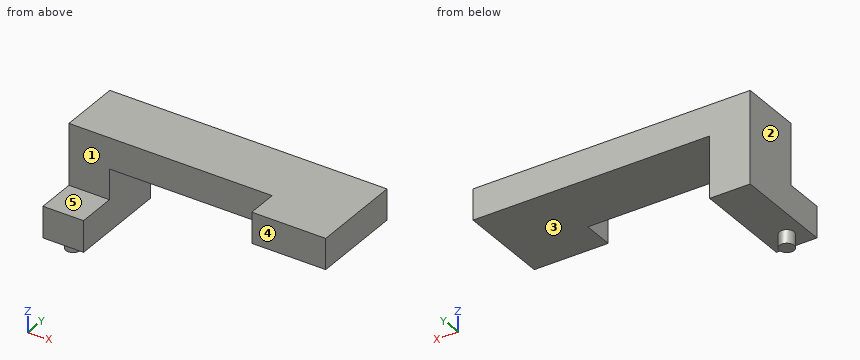
from build123d import *

# Parameters (mm, degrees)
F1_DEPTH = 25.4
F2_W     = 16.7198777199
F2_H     = 12.9023268819
F3_DEPTH = 16.1335784942
F5_W     = 30.4973670125
F5_H     = 12.7
F6_DEPTH = 12.7
F7_R     = 3.015717516
F8_DEPTH = 18.4404


with BuildPart() as f1:
    # F0 (on Front) → F1 (new body)
    with BuildSketch(Plane.XZ):
        Polygon((57.6506801724, -27.7302754164), (-56.6493198276, -27.7302754164), (-56.6493198276, -65.8302754164), (-39.9294421077, -65.8302754164), (-39.9294421077, -40.4302754164), (57.6506801724, -40.4302754164), align=None)
    extrude(amount=F1_DEPTH)

    # F2 (on face) → F3 (join)
    with BuildSketch(Plane.XZ.offset(25.4)):
        with Locations((-48.2893809676, -59.3791119754)):
            Rectangle(F2_W, F2_H)
    extrude(amount=F3_DEPTH)

    # F5 (on face) → F6 (join)
    with BuildSketch(Plane.XZ.offset(25.4)):
        with Locations((42.4019966662, -34.0802754164)):
            Rectangle(F5_W, F5_H)
    extrude(amount=F6_DEPTH)

    # F7 (on face) → F8 (join)
    with BuildSketch(Plane.XY.offset(-52.9279485345)):
        with Locations((-49.315456301, -33.8529422879)):
            Circle(F7_R)
    extrude(amount=-F8_DEPTH)


solid = f1.part
Design review of the part built by this model. Coordinates are the model's own, in mm. Face numbers are marked on the shaded views. A direction names the side the tool comes from. Round coordinates to 2 decimals unless told otherwise and drop trailing zeros. Order: outer loops, then holes, each group sorted by start corner. A loop starts at its lowest first (then second) coordinate and runs counter-clockwise, first axis right, second up. Notation, with made-up numbers: M -36,76 L -22,76 A27 cw -22,93 Z; hole C 0.25,-29.5 d10. An arc over 180 degrees is marked long. Answer as CSV lines item,"result". Start each with the question number.
1) Tool access review of the marked faces 1, 2, 3, 4 and 5: name each direction out of +Z, -Z, +X, -X, +Y, -Y from which nothing blocks a thin tool from reaching the whole face with its end or side.
2) For pin 1 Ø17.5 at (x, y) = (-48, -33.5) entering from +Z; pin 2 Ø8.5 at (x, y) = (-50.5, -10.5) entering from -Z; pin 3 Ø12.5 at (x, z) = (-10, -44.5) entering from -Y; pin 4 Ø7.5 at (y, z) = (-17.5, -53.5) entering from +X, all flat-tipped, find the tip position at first contact; note any pin that passes through.
3) Wall thickness on line 1 along Z through (x, y) = (-4.5, -13.5); line 2 along Z through (x, y) = (-43, -26); line 3 along Y through (x, z) = (-22, -37): over which ranges is each line inside the solid? List them lowest first. Write a range as [from, to].
4) Add section D-D (y = -3). Give the boundary of the cut face in (x, z), then the cut area to 3 significant figures.
5) Add section C-C (z = -60). Give the boundary of the cut face in (x, y), then the cut area to 3 significant figures.
6) Add section A-A (y = -29). Give the boundary of the cut face in (x, z).
7) Add section B-B (x = -43). Give the boundary of the cut face in (y, z).
Resolved:
1,face 1,"+Z, -X, -Y"
1,face 2,"+Z, -Z, -X, +Y, -Y"
1,face 3,"-Z, +X, +Y, -Y"
1,face 4,"+Z, -Z, +X, -X, -Y"
1,face 5,"+Z, +X, -X, -Y"
2,pin 1,"z = -27.73"
2,pin 2,"z = -65.83"
2,pin 3,"y = -25.4"
2,pin 4,"x = -39.93"
3,line 1,"[-40.43, -27.73]"
3,line 2,"[-65.83, -52.93]"
3,line 3,"[-25.4, 0]"
4,outline,"M -56.65,-65.83 L -39.93,-65.83 L -39.93,-40.43 L 57.65,-40.43 L 57.65,-27.73 L -56.65,-27.73 Z"
4,area,"1,880 mm^2"
5,outline,"M -56.65,-41.53 L -39.93,-41.53 L -39.93,0 L -56.65,0 Z"
5,area,"694 mm^2"
6,outline,"M -56.65,-65.83 L -39.93,-65.83 L -39.93,-52.93 L -56.65,-52.93 Z; M 27.15,-40.43 L 57.65,-40.43 L 57.65,-27.73 L 27.15,-27.73 Z"
7,outline,"M -41.53,-65.83 L 0,-65.83 L 0,-27.73 L -25.4,-27.73 L -25.4,-52.93 L -41.53,-52.93 Z"
